Verification items for the finished model (mm, model axes). Face numbers are marked on the shaded views. A direction names the side the tool comes from. Give positions to 0.01 mm unless a question says otherwise; leave off trailing zeros. Write each loop counter-clockwise with the first axis right and the second up, starting at its lowest first coordinate (ties: lowest second). Pieces come first, ordered by that corner, then holes. Notation, with made-up numbers: (12, 32.5) -> (55, 32.5) arc R25 cw to (55, 59.5) -> close; hole circle Ø3 at (20, -37.5). An arc over 180 degrees is marked (long way). Answer as CSV lines item,"result".
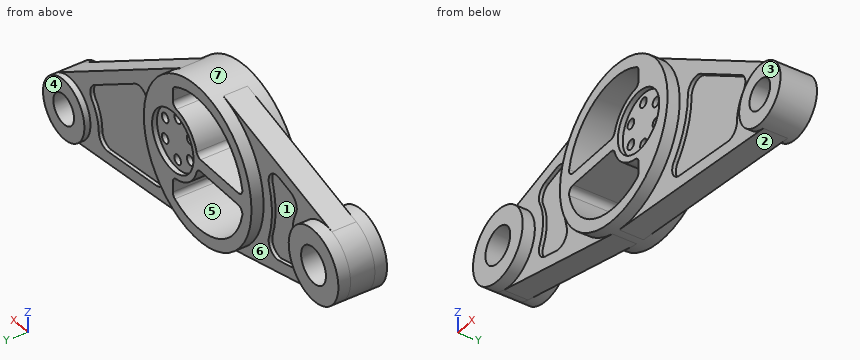
```python
from build123d import *

# Parameters (mm, degrees)
BOSS_EXTRUDE1_DEPTH  = 10
SKETCH2_R            = 65
BOSS_EXTRUDE2_DEPTH  = 20
SKETCH3_R            = 30
BOSS_EXTRUDE3_DEPTH  = 20
SKETCH5_R            = 25
BOSS_EXTRUDE4_DEPTH  = 15
CUT_EXTRUDE1_DEPTH   = 41
SKETCH8_R            = 25
CUT_EXTRUDE3_DEPTH   = 4
SKETCH9_R            = 4
CUT_EXTRUDE4_DEPTH   = 37
CIRPATTERN1_COUNT    = 6
SKETCH10_R           = 15
CUT_EXTRUDE5_DEPTH   = 41
SKETCH11_R           = 12.5
CUT_EXTRUDE6_DEPTH   = 36
CUT_EXTRUDE7_DEPTH   = 3
FILLET1_R            = 10
FILLET1_OF_MIRROR3_R = 10


with BuildPart() as part:
    # Sketch1 → Boss-Extrude1 (new body, symmetric)
    with BuildSketch(Plane(origin=(0, 0, 0), x_dir=(1, 0, 0), z_dir=(0, 1, 0))):
        with BuildLine():
            Line((-147.5, 29.047375), (-16.25, 62.935979))
            ThreePointArc((-16.25, 62.935979), (-12.200915, 63.844637), (-8.102101, 64.493069))
            Line((-8.102101, 64.493069), (166.028479, 86.368652))
            ThreePointArc((166.028479, 86.368652), (192.636987, 70.114129), (182.701893, 40.558823))
            Line((182.701893, 40.558823), (35.248776, -54.612487))
            ThreePointArc((35.248776, -54.612487), (10.371042, -64.167293), (-16.25, -62.935979))
            Line((-16.25, -62.935979), (-147.5, -29.047375))
            ThreePointArc((-147.5, -29.047375), (-170, 0), (-147.5, 29.047375))
        make_face()
    extrude(amount=BOSS_EXTRUDE1_DEPTH, both=True)

    # Sketch2 → Boss-Extrude2 (add, symmetric)
    with BuildSketch(Plane(origin=(0, 0, 0), x_dir=(1, 0, 0), z_dir=(0, 1, 0))):
        with Locations(Location((0, 0, 0), (0, 0, 270))):  # turned: the seam where the file's is
            Circle(SKETCH2_R)
    extrude(amount=BOSS_EXTRUDE2_DEPTH, both=True)

    # Sketch3 → Boss-Extrude3 (add, symmetric)
    with BuildSketch(Plane(origin=(0, 0, 0), x_dir=(1, 0, 0), z_dir=(0, 1, 0))):
        with Locations(Location((-140, 0, 0), (0, 0, 270))):  # turned: the seam where the file's is
            Circle(SKETCH3_R)
    extrude(amount=BOSS_EXTRUDE3_DEPTH, both=True)

    # Sketch5 → Boss-Extrude4 (add, symmetric)
    with BuildSketch(Plane(origin=(0, 0, 0), x_dir=(1, 0, 0), z_dir=(0, 1, 0))):
        with Locations(Location((169.144672, 61.563626, 0), (0, 0, 270))):  # turned: the seam where the file's is
            Circle(SKETCH5_R)
    extrude(amount=BOSS_EXTRUDE4_DEPTH, both=True)

    # Sketch6 → Cut-Extrude1 (cut, through all)
    with BuildSketch(Plane(origin=(0, 20, 0), x_dir=(1, 0, 0), z_dir=(0, 1, 0))):
        with BuildLine():
            Line((-48.989795, 5), (-3.54102, 5))
            ThreePointArc((-3.54102, 5), (-0.552948, 5.991081), (1.250555, 8.571429))
            ThreePointArc((1.250555, 8.571429), (10.395071, 22.707857), (25.714286, 29.6923))
            ThreePointArc((25.714286, 29.6923), (28.779645, 31.367748), (30, 34.641016))
            Line((30, 34.641016), (30, 43.30127))
            ThreePointArc((30, 43.30127), (29.330127, 45.80127), (27.5, 47.631397))
            ThreePointArc((27.5, 47.631397), (-22.573362, 50.154196), (-53.888774, 11))
            ThreePointArc((-53.888774, 11), (-52.862778, 6.837722), (-48.989795, 5))
        make_face()
    cut_extrude1 = extrude(amount=-CUT_EXTRUDE1_DEPTH, mode=Mode.SUBTRACT)

    # Mirror1: Cut-Extrude1 across plane
    add(cut_extrude1.mirror(Plane.XY), mode=Mode.SUBTRACT)

    # Sketch8 → Cut-Extrude3 (cut)
    with BuildSketch(Plane(origin=(0, 20, 0), x_dir=(1, 0, 0), z_dir=(0, 1, 0))):
        with Locations(Location((30, 0, 0), (0, 0, 270))):  # turned: the seam where the file's is
            Circle(SKETCH8_R)
    cut_extrude3 = extrude(amount=-CUT_EXTRUDE3_DEPTH, mode=Mode.SUBTRACT)

    # Mirror2: Cut-Extrude3 across plane
    add(cut_extrude3.mirror(Plane.ZX), mode=Mode.SUBTRACT)

    # Sketch9 → Cut-Extrude4 (cut, through all)
    with BuildSketch(Plane(origin=(0, 16, 0), x_dir=(1, 0, 0), z_dir=(0, 1, 0))):
        with Locations(Location((30, 17.5, 0), (0, 0, 270))):  # turned: the seam where the file's is
            Circle(SKETCH9_R)
    cut_extrude4 = extrude(amount=-CUT_EXTRUDE4_DEPTH, mode=Mode.SUBTRACT)

    # CirPattern1: Cut-Extrude4 ×6 about axis
    cirpattern1_axis = Axis((30, 0, 0), (0, 1, 0))
    for i in range(1, CIRPATTERN1_COUNT):
        add(cut_extrude4.rotate(cirpattern1_axis, i * 360 / CIRPATTERN1_COUNT), mode=Mode.SUBTRACT)

    # Sketch10 → Cut-Extrude5 (cut, through all)
    with BuildSketch(Plane(origin=(0, 20, 0), x_dir=(1, 0, 0), z_dir=(0, 1, 0))):
        with Locations(Location((-140, 0, 0), (0, 0, 270))):  # turned: the seam where the file's is
            Circle(SKETCH10_R)
    extrude(amount=-CUT_EXTRUDE5_DEPTH, mode=Mode.SUBTRACT)

    # Sketch11 → Cut-Extrude6 (cut, through all)
    with BuildSketch(Plane(origin=(0, 15, 0), x_dir=(1, 0, 0), z_dir=(0, 1, 0))):
        with Locations(Location((169.144672, 61.563626, 0), (0, 0, 270))):  # turned: the seam where the file's is
            Circle(SKETCH11_R)
    extrude(amount=-CUT_EXTRUDE6_DEPTH, mode=Mode.SUBTRACT)

    # Sketch12 → Cut-Extrude7 (cut)
    with BuildSketch(Plane(origin=(0, 10, 0), x_dir=(1, 0, 0), z_dir=(0, 1, 0))):
        with BuildLine():
            Line((72.667447, -18.559151), (150.709797, 31.812064))
            ThreePointArc((150.709797, 31.812064), (136.25543, 49.592921), (135.898804, 72.504935))
            Line((135.898804, 72.504935), (43.736902, 60.926869))
            ThreePointArc((43.736902, 60.926869), (70.476947, 25.651511), (72.667447, -18.559151))
        make_face()
        with BuildLine():
            Line((-63.121044, 40.505972), (-111.45898, 28.025171))
            ThreePointArc((-111.45898, 28.025171), (-100, 0), (-111.45898, -28.025171))
            Line((-111.45898, -28.025171), (-63.121044, -40.505972))
            ThreePointArc((-63.121044, -40.505972), (-75, 0), (-63.121044, 40.505972))
        make_face()
    cut_extrude7 = extrude(amount=-CUT_EXTRUDE7_DEPTH, mode=Mode.SUBTRACT)

    # Fillet1
    fillet1_edges = [part.edges().sort_by_distance(p)[0] for p in [
        (-63.121044, 8.5, -40.505972),
        (-63.121044, 8.5, 40.505972),
        (-111.45898, 8.5, 28.025171),
        (-111.45898, 8.5, -28.025171),
        (72.667447, 8.5, 18.559151),
        (43.736902, 8.5, -60.926869),
        (135.898804, 8.5, -72.504935),
        (150.709797, 8.5, -31.812064),
    ]]
    fillet(fillet1_edges, radius=FILLET1_R)

    # Mirror3: Cut-Extrude7 across plane
    add(cut_extrude7.mirror(Plane.ZX), mode=Mode.SUBTRACT)

    # Fillet1 of Mirror3
    fillet1_of_mirror3_edges = [part.edges().sort_by_distance(p)[0] for p in [
        (-63.121044, -8.5, -40.505972),
        (-63.121044, -8.5, 40.505972),
        (-111.45898, -8.5, 28.025171),
        (-111.45898, -8.5, -28.025171),
        (72.667447, -8.5, 18.559151),
        (43.736902, -8.5, -60.926869),
        (135.898804, -8.5, -72.504935),
        (150.709797, -8.5, -31.812064),
    ]]
    fillet(fillet1_of_mirror3_edges, radius=FILLET1_OF_MIRROR3_R)


solid = part.part
```
1) Section check A-A (z = 40). Record the boundary of the cut face in (x, y), and give its area (3 significant figures).
Reported:
outline,"(-105.08, -10) -> (-51.23, -10) -> (-51.23, -20) -> (-37.75, -20) -> (-37.75, 20) -> (-51.23, 20) -> (-51.23, 10) -> (-105.08, 10) -> close; (30, -20) -> (51.23, -20) -> (51.23, -10) -> (57.89, -10) -> (57.89, 10) -> (51.23, 10) -> (51.23, 20) -> (30, 20) -> close"
area,"2,600 mm²"
2) Tool access check on the marked faces 4, 5, 6 and 7. Record the directions out of +Z, -Z, +X, -X, +Y, -Y that give a thin tool (end or side, any length) a straight path to the whole face; none if there is none.
Reported:
face 4,"+Z, -Z, +X, +Y"
face 5,"+Y, -Y"
face 6,"+Y"
face 7,"none"
3) Section check B-B (y = 2.5). State how many separate pieces and enclosed holes the cut face has, and give its area (3 significant figures).
Reported:
separate pieces,"1"
enclosed holes,"10"
area,"25,300 mm²"
4) Section check C-C (x = 119). Record the boundary of the cut face in (y, z), and give its area (3 significant figures).
Reported:
outline,"(-10, -80.46) -> (10, -80.46) -> (10, -70.38) -> (7, -70.38) -> (7, -11.35) -> (10, -11.35) -> (10, 0.56) -> (-10, 0.56) -> (-10, -11.35) -> (-7, -11.35) -> (-7, -70.38) -> (-10, -70.38) -> close"
area,"1,270 mm²"
5) Depth check by flat-ended pin: pin 1 (10 mm diameter, centred on y = 15.5, z = -36, fed in from -X); pin 2 (4 mm diameter, centred on y = -7.5, z = -54, fed in from +X); pin 3 (10 mm diameter, centred on x = -89.5, z = -1.5, fed in from -Y). Enter the tip coordinate at first touch or a pass-through.
Reported:
pin 1,"x = -57.13"
pin 2,"x = 193.52"
pin 3,"y = -7"
6) Scan lines: line 1 along X through (y, z) = (-4.5, 8.75); line 2 along Z through (x, y) = (-7.5, -17.5); line 3 along Z through (x, y) = (3, 12). Record each from-to range of solid material in increasing order.
Reported:
line 1,"-168.7 to -152.18, -127.82 to -53.83, 1.3 to 10.84, 18.84 to 41.16, 49.16 to 106.31"
line 2,"-64.57 to -54.49, -5 to 5, 54.49 to 64.57"
line 3,"-64.93 to -54.92, -13.08 to 13.08, 54.92 to 64.93"
7) Draft check along X on the marked faces 1, 2 and 3. Enter one of: +X half, -X half, draft (parallel to the pull), parting line (faces both ways), or undercut.
Reported:
face 1,"undercut"
face 2,"-X half"
face 3,"draft"
